Here's how the part is built. I have some questions about the finished solid (model axes, mm). A direction names the side the tool comes from. Give positions to 0.01 mm unless a question says otherwise; leave off trailing zeros. Write each loop counter-clockwise with the first axis right and the second up, starting at its lowest first coordinate (ties: lowest second). Pieces come first, ordered by that corner, then holes. Notation, with made-up numbers: (35.5, -16) - (72.5, -16) arc R28 cw to (72.5, 15) - close; hole circle Ø2 at (76, -27.5). An arc over 180 degrees is marked (long way). Write each question's results on one line, items separated by ' | '. Start each with the question number.
Item 1: Suppose I cut it at D-D on z = 3. List the corners of the cut face in (x, y) for me, then the cut area to 3 significant figures.
Item 2: Suppose I cut it at B-B on y = 0. List the corners of the cut face in (x, z) for me, then the cut area to 3 significant figures.
Item 3: Suppose I cut it at A-A on x = 0. List the corners of the cut face in (y, z) for me.
Item 4: Please list where these lines run through material, in increasing order: line 1 along Z through (x, y) = (0.55, -1.9); line 2 along Z through (x, y) = (-1, 0); line 3 along X through (y, z) = (-0.75, 0.5).
Item 5: Suppose I cut it at C-C on z = 10.25. List the corners of the cut face in (x, y) for me, then the cut area to 3 significant figures.
Item 6: Which directions (+Z, -Z, +X, -X, +Y, -Y) give clear straight access to the entire face, cutting with the end or side of a thin tool? Please do faces 1 (the flat face through (-0.3, 0, 0.4)), 2 (the flat face through (1, 1, 1.85)), 3 (the cylindrical face through (1.29, -2.024, 1.037)).
Item 7: We'd pull the mould along X, two halves only. Please class faces 4 (the flat face through (-1, 0, 0)), 5 (the flat face through (0.3, 0, 0.4)), 6 (the cylindrical face through (-0.18, 0.83, 9.4)): +X half, -X half, draft (parallel to the pull), parting line (faces both ways), or undercut.
Item 8: Will these pins go through, and if not, where does the flat tip stop? P1, Ø1.5, axis at y = -1.5, z = 7.5, coming from the +X side; P2, Ø1.5, axis at x = 1, y = 2, coming from the +Z side; P3, Ø1.5, axis at x = 1, z = 2, coming from the -Y side.
```python
from build123d import *

# Parameters (mm, degrees)
F2_SIZE  = 0.25
F4_DEPTH = 0.9
F5_SIZE  = 0.2


with BuildPart() as f1:
    # F0 (on Front) → F1 (revolve)
    with BuildSketch(Plane.XZ):
        Polygon((0, 11.2), (0, 0), (2.4, 0), (2.4, 1.85), (1.25, 1.85), (1.25, 7.8), (0.85, 7.8), (0.85, 11.2), align=None)
    revolve(axis=Axis((0, 0, 5.6), (0, 0, -1)))

    # F2
    f2_edges = [f1.edges().sort_by_distance(p)[0] for p in [
        (-0.85, 0, 11.2),
    ]]
    chamfer(f2_edges, length=F2_SIZE)

    # F3 (on face) → F4 (cut)
    with BuildSketch(Plane(origin=(0, 0, 0), x_dir=(1, 0, 0), z_dir=(0, 0, -1))):
        with BuildLine():
            ThreePointArc((0.3, 2.38117618), (0, 2.4), (-0.3, 2.38117618))
            Line((-0.3, 2.38117618), (-0.3, -2.38117618))
            ThreePointArc((-0.3, -2.38117618), (0, -2.4), (0.3, -2.38117618))
            Line((0.3, -2.38117618), (0.3, 2.38117618))
        make_face()
    extrude(amount=-F4_DEPTH, mode=Mode.SUBTRACT)

    # F5
    f5_edges = [f1.edges().sort_by_distance(p)[0] for p in [
        (1.8, 1.587451, 0),
        (1.8, -1.587451, 0),
        (-2.4, 0, 0),
    ]]
    chamfer(f5_edges, length=F5_SIZE)


solid = f1.part
```
Checked values:
1) outline: circle Ø2.5 at (0, 0) | area: 4.91 mm^2
2) outline: (-2.4, 0.2) - (-2.2, 0) - (-0.3, 0) - (-0.3, 0.9) - (0.3, 0.9) - (0.3, 0) - (2.2, 0) - (2.4, 0.2) - (2.4, 1.85) - (1.25, 1.85) - (1.25, 7.8) - (0.85, 7.8) - (0.85, 10.95) - (0.6, 11.2) - (-0.6, 11.2) - (-0.85, 10.95) - (-0.85, 7.8) - (-1.25, 7.8) - (-1.25, 1.85) - (-2.4, 1.85) - close | area: 28.9 mm^2
3) outline: (-2.4, 0.9) - (2.4, 0.9) - (2.4, 1.85) - (1.25, 1.85) - (1.25, 7.8) - (0.85, 7.8) - (0.85, 10.95) - (0.6, 11.2) - (-0.6, 11.2) - (-0.85, 10.95) - (-0.85, 7.8) - (-1.25, 7.8) - (-1.25, 1.85) - (-2.4, 1.85) - close
4) line 1: z = 0 to 1.85 | line 2: z = 0 to 7.8 | line 3: x = -2.28 to -0.3, 0.3 to 2.28
5) outline: circle Ø1.7 at (0, 0) | area: 2.27 mm^2
6) face 1: -Z, +Y, -Y | face 2: +Z | face 3: +Z, -Z
7) face 4: draft | face 5: undercut | face 6: parting line
8) P1: stops at x = 1 | P2: stops at z = 1.85 | P3: stops at y = -2.39
